Part model, mm, in its own coordinate system. A direction names the side the tool comes from. Give positions to 0.01 mm unless a question says otherwise; leave off trailing zeros. Order: outer loops, then holes, each group sorted by start corner. A loop starts at its lowest first (then second) coordinate and runs counter-clockwise, first axis right, second up. Notation, with made-up numbers: (51, 87) - (93, 87) arc R11 cw to (93, 98) - close; hole circle Ø4 at (51.25, 63). An arc over 180 degrees is marked (long way). One line per item, written item: value.
```python
from build123d import *

# Parameters (mm, degrees)
ESQUISSE1_R             = 1.25
BOSS_EXTRU_1_DEPTH      = 8
TROU_TARAUD_M3_D        = 3.4
ESQUISSE4_R             = 1.6
ENL_V_MAT_EXTRU_1_DEPTH = 9
ESQUISSE5_R             = 4
ENL_V_MAT_EXTRU_2_DEPTH = 5


with BuildPart() as part:
    # Esquisse1 → Boss.-Extru.1 (new body)
    with BuildSketch(Plane.XY):
        with BuildLine():
            Line((2.96841177, 10.030192742), (146.96841177, 10.030192742))
            ThreePointArc((146.96841177, 10.030192742), (149.089732114, 10.908872398), (149.96841177, 13.030192742))
            Line((149.96841177, 13.030192742), (149.96841177, 97.09690847))
            ThreePointArc((149.96841177, 97.09690847), (149.301594422, 98.982712998), (147.597572626, 100.030192742))
            Line((147.597572626, 100.030192742), (2.96841177, 100.030192742))
            ThreePointArc((2.96841177, 100.030192742), (0.847091427, 99.151513085), (-0.03158823, 97.030192742))
            Line((-0.03158823, 97.030192742), (-0.03158823, 13.030192742))
            ThreePointArc((-0.03158823, 13.030192742), (0.847091427, 10.908872398), (2.96841177, 10.030192742))
        make_face()
        with Locations((12.96841177, 97.530192742)):
            Circle(ESQUISSE1_R, mode=Mode.SUBTRACT)
        with Locations((74.96841177, 97.530192742)):
            Circle(ESQUISSE1_R, mode=Mode.SUBTRACT)
        with Locations((136.96841177, 97.530192742)):
            Circle(ESQUISSE1_R, mode=Mode.SUBTRACT)
        with Locations((12.96841177, 55.030192742)):
            Circle(ESQUISSE1_R, mode=Mode.SUBTRACT)
        with Locations((74.96841177, 55.030192742)):
            Circle(ESQUISSE1_R, mode=Mode.SUBTRACT)
        with Locations((136.96841177, 55.030192742)):
            Circle(ESQUISSE1_R, mode=Mode.SUBTRACT)
        with Locations((136.96841177, 12.530192742)):
            Circle(ESQUISSE1_R, mode=Mode.SUBTRACT)
        with Locations((74.96841177, 12.530192742)):
            Circle(ESQUISSE1_R, mode=Mode.SUBTRACT)
        with Locations((12.96841177, 12.530192742)):
            Circle(ESQUISSE1_R, mode=Mode.SUBTRACT)
    extrude(amount=BOSS_EXTRU_1_DEPTH)

    # Trou taraudé M3 (through all)
    with Locations(Plane.XY.offset(8)):
        with Locations((12.96841177, 97.530192742), (12.96841177, 55.030192742), (12.96841177, 12.530192742), (74.96841177, 12.530192742), (74.96841177, 55.030192742), (74.96841177, 97.530192742), (136.96841177, 97.530192742), (136.96841177, 55.030192742), (136.96841177, 12.530192742)):
            Hole(TROU_TARAUD_M3_D / 2)

    # Esquisse4 → Enlèv. mat.-Extru.1 (cut, through all)
    with BuildSketch(Plane.XY.offset(8)):
        with Locations((119.96841177, 95.030192742)):
            Circle(ESQUISSE4_R)
        with Locations((49.96841177, 95.030192742)):
            Circle(ESQUISSE4_R)
        with Locations((4.96841177, 76.55605286)):
            Circle(ESQUISSE4_R)
        with Locations((4.96841177, 34.250278271)):
            Circle(ESQUISSE4_R)
        with Locations((49.96841177, 15.030192742)):
            Circle(ESQUISSE4_R)
        with Locations((119.96841177, 15.030192742)):
            Circle(ESQUISSE4_R)
        with Locations((64.96841177, 55.030192742)):
            Circle(ESQUISSE4_R)
        with Locations((124.96841177, 55.030192742)):
            Circle(ESQUISSE4_R)
    extrude(amount=-ENL_V_MAT_EXTRU_1_DEPTH, mode=Mode.SUBTRACT)

    # Esquisse5 → Enlèv. mat.-Extru.2 (cut)
    with BuildSketch(Plane.XY.offset(8)):
        with Locations((49.96841177, 95.030192742)):
            Circle(ESQUISSE5_R)
        with Locations((119.96841177, 95.030192742)):
            Circle(ESQUISSE5_R)
        with Locations((124.96841177, 55.030192742)):
            Circle(ESQUISSE5_R)
        with Locations((64.96841177, 55.030192742)):
            Circle(ESQUISSE5_R)
        with Locations((4.96841177, 76.55605286)):
            Circle(ESQUISSE5_R)
        with Locations((4.96841177, 34.250278271)):
            Circle(ESQUISSE5_R)
        with Locations((49.96841177, 15.030192742)):
            Circle(ESQUISSE5_R)
        with Locations((119.96841177, 15.030192742)):
            Circle(ESQUISSE5_R)
    extrude(amount=-ENL_V_MAT_EXTRU_2_DEPTH, mode=Mode.SUBTRACT)


solid = part.part
```
1) Cut at A-A, the plane x = 65. Give the cut face in (y, z), then the cut area to 3 significant figures.
Outcome:
outline: (10.03, 0) - (53.43, 0) - (53.43, 3) - (51.03, 3) - (51.03, 8) - (10.03, 8) - close; (56.63, 0) - (100.03, 0) - (100.03, 8) - (59.03, 8) - (59.03, 3) - (56.63, 3) - close
area: 670 mm^2
2) Mould opens along X. For faces 3 (the cylindrical face through (0.824, 10.932, 3.944)), 4 (the cylindrical face through (136.184, 96.022, 3.944)), 5 (the flat face through (74, 66, 8)), 6 (the cylindrical face through (5.83, 35.6, 1.52)) say: released by +X, released by -X, zero draft, split by the parting line, or undercut.
Outcome:
face 3: released by -X
face 4: undercut
face 5: zero draft
face 6: undercut
3) Which spindle directions (+Z, -Z, +X, -X, +Y, -Y) get a long thin tool onto all of the face, cutting with end or side? Do faces 1 (the cylindrical face through (121.446, 14.417, 1.521)), 2 (the flat face through (7, 77, 3)). Say none if no direction does.
Outcome:
face 1: +Z, -Z
face 2: +Z
4) Pin check, flat tips, straight feed: pin 1 (13 mm diameter, centred on x = 4.97, y = 76.56, fed in from -Z); pin 2 (3 mm diameter, centred on x = 12.97, y = 97.53, fed in from -Z); pin 3 (5 mm diameter, centred on x = 4.97, y = 34.25, fed in from +Z). Stop position of each tip, or through.
Outcome:
pin 1: stops at z = 0
pin 2: passes through
pin 3: stops at z = 3
5) Drill centre lines: line 1 along X through (y, z) = (15, 4.75); line 2 along X through (y, z) = (34, 3.25); line 3 along X through (y, z) = (57, 5). Where is each one in solid material? Low to high. Write a range as from..to.
Outcome:
line 1: x = -0.03..45.97, 53.97..115.97, 123.97..149.97
line 2: x = -0.03..0.98, 8.96..149.97
line 3: x = -0.03..61.49, 68.45..121.49, 128.45..149.97
6) Cut at B-B, the plane z = 6. Give the number of separate pieces and of enclosed holes in the cut face, then the cut area to 3 significant figures.
Outcome:
separate pieces: 1
enclosed holes: 17
area: 13,000 mm^2
